Read the model definition and answer for the solid it produces. Units are mm, in the model's axes. Face numbers are marked on the shaded views. Coordinates: 2 decimals unless noted, no trailing zeros. Order: outer loops, then holes, each group sorted by start corner. A loop starts at its lowest first (then second) coordinate and runs counter-clockwise, first axis right, second up. Notation, with made-up numbers: M 87,-8.75 L 119,-8.75 A26 ccw 119,29.25 Z; hole C -23.75,36.5 d1. An arc over 180 degrees is marked long. Write each question's results on one line, items separated by ' | '.
```python
from build123d import *

# Parameters (mm, degrees)
SKETCH_1_W          = 4
SKETCH_1_H          = 4
EXTRUDE_1_DEPTH     = 30
SKETCH_3_W          = 2
SKETCH_3_H          = 4
CUT_EXTRUDE_1_DEPTH = 2
SKETCH_4_W          = 4
SKETCH_4_H          = 2
CUT_EXTRUDE_2_DEPTH = 4
SKETCH_5_W          = 2
SKETCH_5_H          = 2
CUT_EXTRUDE_3_DEPTH = 2


with BuildPart() as part:
    # 草圖1 → 填料-伸長1 (new body)
    with BuildSketch(Plane.XY):
        Rectangle(SKETCH_1_W, SKETCH_1_H)
    extrude(amount=EXTRUDE_1_DEPTH)

    # 草圖3 → 除料-伸長1 (cut)
    with BuildSketch(Plane.ZY.offset(2)):
        with Locations((12, 0)):
            Rectangle(SKETCH_3_W, SKETCH_3_H)
    extrude(amount=-CUT_EXTRUDE_1_DEPTH, mode=Mode.SUBTRACT)

    # 草圖4 → 除料-伸長2 (cut)
    with BuildSketch(Plane.ZY.offset(2)):
        with Locations((15, 1)):
            Rectangle(SKETCH_4_W, SKETCH_4_H)
    extrude(amount=-CUT_EXTRUDE_2_DEPTH, mode=Mode.SUBTRACT)

    # 草圖5 → 除料-伸長3 (cut)
    with BuildSketch(Plane.ZY.offset(2)):
        with Locations((14, -1)):
            Rectangle(SKETCH_5_W, SKETCH_5_H)
    extrude(amount=-CUT_EXTRUDE_3_DEPTH, mode=Mode.SUBTRACT)


solid = part.part
```
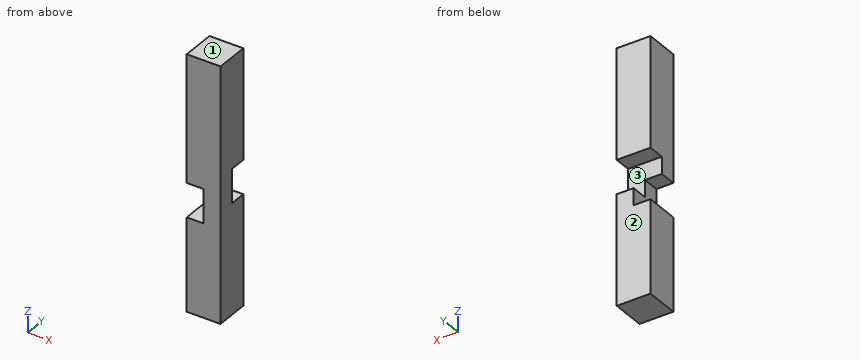
(1) The part is cut by section D-D, the plane y = -1.65. Write down the section's boundary in (x, z), then the cut area to 3 significant figures.
Conclusion:
outline: M -2,0 L 2,0 L 2,30 L -2,30 L -2,15 L 0,15 L 0,11 L -2,11 Z | area: 112 mm²
(2) The mould has two halves that part along Z. Classify the marked faces 1, 2 and 3: pulls with the +Z half, pulls with the -Z half, needs draft (parallel to the pull), parting line crosses it, or undercut.
Conclusion:
face 1: pulls with the +Z half | face 2: needs draft | face 3: undercut
(3) Straight lines are drawn through the part: line 1 (Z direction, x = -0.4, y = -0.95); line 2 (Z direction, x = -1.75, y = 1.05); line 3 (X direction, y = -0.9, z = 11.75). For each, find the intervals that lie inside material, in ascending order.
Conclusion:
line 1: 0 to 11, 15 to 30 | line 2: 0 to 11, 17 to 30 | line 3: 0 to 2
(4) The part is cut by section B-B, the plane y = 1.5. Write down the section's boundary in (x, z).
Conclusion:
outline: M -2,0 L 2,0 L 2,13 L 0,13 L 0,11 L -2,11 Z; M -2,17 L 2,17 L 2,30 L -2,30 Z
(5) The part is cut by section A-A, the plane x = -0.9. Write down the section's boundary in (y, z), then the cut area to 3 significant figures.
Conclusion:
outline: M -2,0 L 2,0 L 2,11 L -2,11 Z; M -2,15 L 0,15 L 0,17 L 2,17 L 2,30 L -2,30 Z | area: 100 mm²
(6) The part is cut by section C-C, the plane x = 1.7. Write down the section's boundary in (y, z).
Conclusion:
outline: M -2,0 L 2,0 L 2,13 L 0,13 L 0,17 L 2,17 L 2,30 L -2,30 Z
